from build123d import *

# Parameters (mm, degrees)
SKETCH_1_W                   = 65
SKETCH_1_H                   = 30
EXTRUDE_1_DEPTH              = 8
HOLE_WIZARD_M6_1_D           = 6.6
HOLE_WIZARD_M6_1_DEPTH       = 20
HOLE_WIZARD_M6_1_CSINK_D     = 6.65
HOLE_WIZARD_M6_1_CSINK_ANGLE = 90
HOLE_WIZARD_M6_1_TIP         = 1.982840043
HOLE_WIZARD_M6_2_D           = 12.5
HOLE_WIZARD_M6_2_DEPTH       = 20
HOLE_WIZARD_M6_2_CSINK_D     = 12.6
HOLE_WIZARD_M6_2_CSINK_ANGLE = 90
HOLE_WIZARD_M6_2_TIP         = 3.755378869


with BuildPart() as part:
    # 草图1 → 凸台-拉伸1 (new body)
    with BuildSketch(Plane.XY):
        Rectangle(SKETCH_1_W, SKETCH_1_H)
    extrude(amount=EXTRUDE_1_DEPTH)

    # M6 间隙槽口1
    with Locations(Plane.XY.offset(8)):
        with Locations((-17.5, 0)):
            CounterSinkHole(HOLE_WIZARD_M6_1_D / 2, HOLE_WIZARD_M6_1_CSINK_D / 2, depth=HOLE_WIZARD_M6_1_DEPTH, counter_sink_angle=HOLE_WIZARD_M6_1_CSINK_ANGLE)
            with Locations((0, 0, -(HOLE_WIZARD_M6_1_DEPTH + HOLE_WIZARD_M6_1_TIP / 2))):  # 118° drill point
                Cone(0, HOLE_WIZARD_M6_1_D / 2, HOLE_WIZARD_M6_1_TIP, mode=Mode.SUBTRACT)

    # M6 间隙槽口2
    with Locations(Plane.XY.offset(8)):
        with Locations((17.5, 0)):
            CounterSinkHole(HOLE_WIZARD_M6_2_D / 2, HOLE_WIZARD_M6_2_CSINK_D / 2, depth=HOLE_WIZARD_M6_2_DEPTH, counter_sink_angle=HOLE_WIZARD_M6_2_CSINK_ANGLE)
            with Locations((0, 0, -(HOLE_WIZARD_M6_2_DEPTH + HOLE_WIZARD_M6_2_TIP / 2))):  # 118° drill point
                Cone(0, HOLE_WIZARD_M6_2_D / 2, HOLE_WIZARD_M6_2_TIP, mode=Mode.SUBTRACT)


solid = part.part
Here's how the part is built. I have some questions about the finished solid (model axes, mm). Round coordinates to 2 decimals unless told otherwise and drop trailing zeros. Order: outer loops, then holes, each group sorted by start corner. A loop starts at its lowest first (then second) coordinate and runs counter-clockwise, first axis right, second up. Notation, with made-up numbers: M -14,48 L 35,48 A22 cw 35,65 Z; hole C 73.5,65.5 d11. An arc over 180 degrees is marked long. Return JSON: item names as keys, results as strings. Group by question number.
1. Please list where these lines run through material, in increasing order: probe 1 along X at (y, z) = (-0.25, 1.5) (3 decimals); probe 2 along X at (y, z) = (-2.5, 6.75); probe 3 along Y at (x, z) = (17.5, 2).
2. If we mould it in two halves opening along Y, with no side actions, what happens to faces 1 (the face through (22.46, -3.8, 3.92)), 2 (the face through (0, -15, 4)), 3 (the face through (0, 0, 0)), 4 (the face through (-15.07, 2.23, 3.93))? For each: pulls with the +Y half, pulls with the -Y half, needs draft (parallel to the pull), parting line crosses it, or undercut.
3. If we section it at C-C on x = 17.5: List the corners of the cut face in (y, z) for me.
4. If we section it at D-D on z = 4.5: List the corners of the cut face in (x, y) for me.
5. If we section it at A-A on x = -17.5: List the corners of the cut face in (y, z) for me (3 decimals), then the cut area to 3 significant figures.
6. If we section it at B-B on y = 0: List the corners of the cut face in (x, z) for me (3 decimals), then the cut area to 3 significant figures.
7. I'm going to push a flat-ended pin straight in: pin 1 Ø5 at (x, y) = (21, 9.5) entering from -Z. Where does the tip first touch, or does it pass through?
Reply:
{
 "1": {"probe 1": "-32.5 to -20.791, -14.209 to 11.255, 23.745 to 32.5", "probe 2": "-32.5 to -19.65, -15.35 to 11.77, 23.23 to 32.5", "probe 3": "-15 to -6.25, 6.25 to 15"},
 "2": {"face 1": "undercut", "face 2": "pulls with the -Y half", "face 3": "needs draft", "face 4": "undercut"},
 "3": {"outline": "M -15,0 L -6.25,0 L -6.25,7.95 L -6.3,8 L -15,8 Z; M 6.25,0 L 15,0 L 15,8 L 6.3,8 L 6.25,7.95 Z"},
 "4": {"outline": "M -32.5,-15 L 32.5,-15 L 32.5,15 L -32.5,15 Z; hole C -17.5,0 d6.6; hole C 17.5,0 d12.5"},
 "5": {"outline": "M -15,0 L -3.3,0 L -3.3,7.975 L -3.325,8 L -15,8 Z; M 3.3,0 L 15,0 L 15,8 L 3.325,8 L 3.3,7.975 Z", "area": "187 mm^2"},
 "6": {"outline": "M -32.5,0 L -20.8,0 L -20.8,7.975 L -20.825,8 L -32.5,8 Z; M -14.2,0 L 11.25,0 L 11.25,7.95 L 11.2,8 L -14.175,8 L -14.2,7.975 Z; M 23.75,0 L 32.5,0 L 32.5,8 L 23.8,8 L 23.75,7.95 Z", "area": "367 mm^2"},
 "7": {"pin 1": "z = 0"}
}
